```python
from build123d import *

# Parameters (mm, degrees)
SKETCH_1_R               = 29
EXTRUDE_1_DEPTH          = 4
CUT_EXTRUDE_1_DEPTH      = 42.206795556
CUT_EXTRUDE_1_DEPTH_BACK = 42.206795556
SKETCH_2_R               = 15
EXTRUDE_START            = -5
SKETCH_4_R               = 4
EXTRUDE_3_DEPTH          = 6.5
PATTERN_CIRCULAR_1_COUNT = 4
SKETCH_5_R               = 2.5
CUT_EXTRUDE_2_DEPTH      = 4.5
PATTERN_CIRCULAR_2_COUNT = 4
SKETCH_7_R               = 2.5
CUT_EXTRUDE_3_DEPTH      = 42.31585652
SKETCH_8_R               = 3.5
CUT_EXTRUDE_4_DEPTH      = 2
PATTERN_CIRCULAR_3_COUNT = 4


with BuildPart() as part:
    # 草图1 → 凸台-拉伸1 (new body)
    with BuildSketch(Plane(origin=(0, 0, 0), x_dir=(0, 0, -1), z_dir=(1, 0, 0))):
        Circle(SKETCH_1_R)
    extrude(amount=EXTRUDE_1_DEPTH)

    # 草图2 → 切除-拉伸1 (cut, two sides: drawn at the far end of the back side and taken through both)
    with BuildSketch(Plane(origin=(4, 0, 0), x_dir=(0, 0, -1), z_dir=(1, 0, 0)).offset(-CUT_EXTRUDE_1_DEPTH_BACK)):
        Circle(SKETCH_2_R)
    extrude(amount=CUT_EXTRUDE_1_DEPTH + CUT_EXTRUDE_1_DEPTH_BACK, mode=Mode.SUBTRACT)

    # 草图4 → 凸台-拉伸3 (add)
    with BuildSketch(Plane(origin=(4, 0, 0), x_dir=(0, 0, -1), z_dir=(1, 0, 0)).offset(EXTRUDE_START)):
        with Locations((0, 22)):
            Circle(SKETCH_4_R)
    extrude_3 = extrude(amount=EXTRUDE_3_DEPTH)

    # 阵列(圆周)1: 凸台-拉伸3 ×4 about axis
    pattern_circular_1_axis = Axis((0, 0, 0), (1, 0, 0))
    for i in range(1, PATTERN_CIRCULAR_1_COUNT):
        add(extrude_3.rotate(pattern_circular_1_axis, i * 360 / PATTERN_CIRCULAR_1_COUNT))

    # 草图5 → 切除-拉伸2 (cut)
    with BuildSketch(Plane.ZY.offset(1)):
        with Locations((0, 22)):
            Circle(SKETCH_5_R)
    cut_extrude_2 = extrude(amount=-CUT_EXTRUDE_2_DEPTH, mode=Mode.SUBTRACT)

    # 阵列(圆周)2: 切除-拉伸2 ×4 about axis
    pattern_circular_2_axis = Axis((0, 0, 0), (1, 0, 0))
    for i in range(1, PATTERN_CIRCULAR_2_COUNT):
        add(cut_extrude_2.rotate(pattern_circular_2_axis, i * 360 / PATTERN_CIRCULAR_2_COUNT), mode=Mode.SUBTRACT)

    # 草图7 → 切除-拉伸3 (cut, through all)
    with BuildSketch(Plane(origin=(4, 0, 0), x_dir=(0, 0, -1), z_dir=(1, 0, 0))):
        with Locations((-15.556349186, 15.556349186)):
            Circle(SKETCH_7_R)
    cut_extrude_3 = extrude(amount=-CUT_EXTRUDE_3_DEPTH, mode=Mode.SUBTRACT)

    # 草图8 → 切除-拉伸4 (cut)
    with BuildSketch(Plane(origin=(4, 0, 0), x_dir=(0, 0, -1), z_dir=(1, 0, 0))):
        with Locations((-15.556349186, 15.556349186)):
            Circle(SKETCH_8_R)
    cut_extrude_4 = extrude(amount=-CUT_EXTRUDE_4_DEPTH, mode=Mode.SUBTRACT)

    # 阵列(圆周)3: 切除-拉伸3, 切除-拉伸4 ×4 about axis
    pattern_circular_3_axis = Axis((0, 0, 0), (1, 0, 0))
    add([cut_extrude_3.rotate(pattern_circular_3_axis, i * 360 / PATTERN_CIRCULAR_3_COUNT) for i in range(1, PATTERN_CIRCULAR_3_COUNT)], mode=Mode.SUBTRACT)
    add([cut_extrude_4.rotate(pattern_circular_3_axis, i * 360 / PATTERN_CIRCULAR_3_COUNT) for i in range(1, PATTERN_CIRCULAR_3_COUNT)], mode=Mode.SUBTRACT)


solid = part.part
```
Here's how the part is built. I have some questions about the finished solid (model axes, mm). A direction names the side the tool comes from. Coordinates: 2 decimals unless noted, no trailing zeros. Order: outer loops, then holes, each group sorted by start corner. A loop starts at its lowest first (then second) coordinate and runs counter-clockwise, first axis right, second up.
1) Imagine slicing it at D-D on z = 17. List the corners of the cut face in (x, y) for me, and give its area (3 significant figures).
2) Which directions (+Z, -Z, +X, -X, +Y, -Y) give clear straight access to the entire face, cutting with the end or side of a thin tool? Please do faces 4 (the face through (3.014, 18.334, -13.427)), 5 (the face through (1.014, 17.399, -17.246)), 6 (the face through (0, -12, -12)).
3) Imagine slicing it at C-C on x = 1.25. State how many separate pieces and enclosed holes the cut face has, and give its area (3 significant figures).
4) Will these pins go through, and if not, where does the flat tip stop? pin 1 (2.5 mm diameter, centred on y = 0.5, z = 22, fed in from -X); pin 2 (5.5 mm diameter, centred on y = -17, z = 17, fed in from +X); pin 3 (1.5 mm diameter, centred on x = 3, y = 4.5, fed in from -Z).
5) We'd pull the mould along Z, two halves only. Please class faces 1 (the face through (-0.507, -25.966, -0.521)), 2 (the face through (-1, 24, -2)), 3 (the face through (3.014, -13.427, -18.334)): +Z half, -Z half, draft (parallel to the pull), parting line (faces both ways), or undercut.
6) I need wall thicknesses on line 1 (Y direction, x = 1.75, z = 0); line 2 (Z direction, x = 1.25, y = 1.5); line 3 (Z direction, x = 3.75, y = -16). Which ranges of each line are inside material? Lowest first, please.
Response values:
1. outline: (0, -23.49) - (4, -23.49) - (4, -18.74) - (2, -18.74) - (2, -17.6) - (0, -17.6) - close; (0, -13.52) - (2, -13.52) - (2, -12.37) - (4, -12.37) - (4, 12.37) - (2, 12.37) - (2, 13.52) - (0, 13.52) - close; (0, 17.6) - (2, 17.6) - (2, 18.74) - (4, 18.74) - (4, 23.49) - (0, 23.49) - close
1. area: 146 mm2
2. face 4: +X
2. face 5: +X, -X
2. face 6: -X
3. separate pieces: 1
3. enclosed holes: 9
3. area: 1,780 mm2
4. pin 1: stops at x = 3.5
4. pin 2: stops at x = 4
4. pin 3: stops at z = -28.76
5. face 1: parting line
5. face 2: draft
5. face 3: undercut
6. line 1: y = -29 to -24.5, -19.5 to -15, 15 to 19.5, 24.5 to 29
6. line 2: z = -28.96 to -24, -20 to -14.92, 14.92 to 20, 24 to 28.96
6. line 3: z = -24.19 to -19.03, -12.08 to 12.08, 19.03 to 24.19
